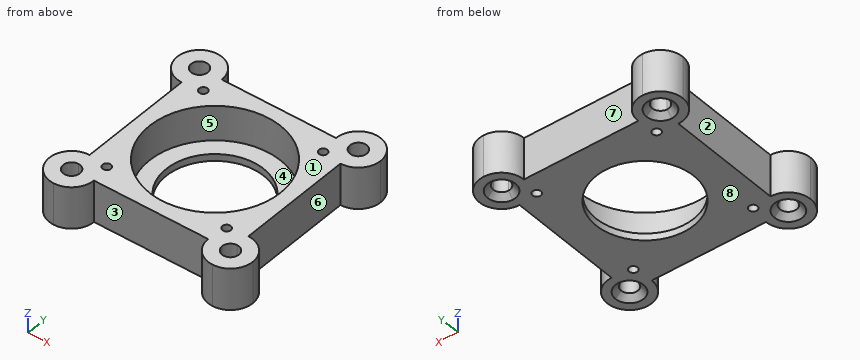
```python
from build123d import *

# Parameters (mm, degrees)
F0_R     = 1.5
F0_R_2   = 23.5
F1_DEPTH = 15
F0_R_3   = 17.5
F2_DEPTH = 2.5
F3_SIZE  = 2


# Not quite as in the source:
# - a feature names something its author has since deleted; it is built from what else it names


with BuildPart() as f1:
    # F0 (on Top) → F1 (new body)
    with BuildSketch(Plane.XY):
        with BuildLine():
            Line((-28.5, 25.5), (-28.5, 20.5))
            ThreePointArc((-28.5, 20.5), (-22.8431457505, 22.8431457505), (-20.5, 28.5))
            Line((-20.5, 28.5), (-25.5, 28.5))
            ThreePointArc((-25.5, 28.5), (-26.3786796564, 26.3786796564), (-28.5, 25.5))
        make_face()
        with BuildLine():
            Line((-20.5, -28.5), (20.5, -28.5))
            ThreePointArc((20.5, -28.5), (22.8431457505, -22.8431457505), (28.5, -20.5))
            Line((28.5, -20.5), (28.5, 20.5))
            ThreePointArc((28.5, 20.5), (22.8431457505, 22.8431457505), (20.5, 28.5))
            Line((20.5, 28.5), (-20.5, 28.5))
            ThreePointArc((-20.5, 28.5), (-22.8431457505, 22.8431457505), (-28.5, 20.5))
            Line((-28.5, 20.5), (-28.5, -20.5))
            ThreePointArc((-28.5, -20.5), (-22.8431457505, -22.8431457505), (-20.5, -28.5))
        make_face()
        with Locations((-21.5, -21.5)):
            Circle(F0_R, mode=Mode.SUBTRACT)
        with Locations((21.5, -21.5)):
            Circle(F0_R, mode=Mode.SUBTRACT)
        with Locations((-21.5, 21.5)):
            Circle(F0_R, mode=Mode.SUBTRACT)
        Circle(F0_R_2, mode=Mode.SUBTRACT)
        with Locations((21.5, 21.5)):
            Circle(F0_R, mode=Mode.SUBTRACT)
        with BuildLine():
            ThreePointArc((20.5, 28.5), (22.8431457505, 22.8431457505), (28.5, 20.5))
            Line((28.5, 20.5), (28.5, 25.5))
            ThreePointArc((28.5, 25.5), (26.3786796564, 26.3786796564), (25.5, 28.5))
            Line((25.5, 28.5), (20.5, 28.5))
        make_face()
        with BuildLine():
            ThreePointArc((28.5, 20.5), (34.1568542495, 22.8431457505), (36.5, 28.5))
            ThreePointArc((36.5, 28.5), (34.1568542495, 34.1568542495), (28.5, 36.5))
            ThreePointArc((28.5, 36.5), (22.8431457505, 34.1568542495), (20.5, 28.5))
            Line((20.5, 28.5), (25.5, 28.5))
            ThreePointArc((25.5, 28.5), (28.5, 31.5), (31.5, 28.5))
            ThreePointArc((31.5, 28.5), (30.6213203436, 26.3786796564), (28.5, 25.5))
            Line((28.5, 25.5), (28.5, 20.5))
        make_face()
        with BuildLine():
            ThreePointArc((20.5, -28.5), (22.8431457505, -34.1568542495), (28.5, -36.5))
            ThreePointArc((28.5, -36.5), (34.1568542495, -34.1568542495), (36.5, -28.5))
            ThreePointArc((36.5, -28.5), (34.1568542495, -22.8431457505), (28.5, -20.5))
            Line((28.5, -20.5), (28.5, -25.5))
            ThreePointArc((28.5, -25.5), (30.6213203436, -26.3786796564), (31.5, -28.5))
            ThreePointArc((31.5, -28.5), (28.5, -31.5), (25.5, -28.5))
            Line((25.5, -28.5), (20.5, -28.5))
        make_face()
        with BuildLine():
            ThreePointArc((28.5, -20.5), (22.8431457505, -22.8431457505), (20.5, -28.5))
            Line((20.5, -28.5), (25.5, -28.5))
            ThreePointArc((25.5, -28.5), (26.3786796564, -26.3786796564), (28.5, -25.5))
            Line((28.5, -25.5), (28.5, -20.5))
        make_face()
        with BuildLine():
            Line((-25.5, -28.5), (-20.5, -28.5))
            ThreePointArc((-20.5, -28.5), (-22.8431457505, -22.8431457505), (-28.5, -20.5))
            Line((-28.5, -20.5), (-28.5, -25.5))
            ThreePointArc((-28.5, -25.5), (-26.3786796564, -26.3786796564), (-25.5, -28.5))
        make_face()
        with BuildLine():
            ThreePointArc((-36.5, -28.5), (-34.1568542495, -34.1568542495), (-28.5, -36.5))
            ThreePointArc((-28.5, -36.5), (-22.8431457505, -34.1568542495), (-20.5, -28.5))
            Line((-20.5, -28.5), (-25.5, -28.5))
            ThreePointArc((-25.5, -28.5), (-30.6213203436, -30.6213203436), (-28.5, -25.5))
            Line((-28.5, -25.5), (-28.5, -20.5))
            ThreePointArc((-28.5, -20.5), (-34.1568542495, -22.8431457505), (-36.5, -28.5))
        make_face()
        with BuildLine():
            ThreePointArc((-28.4999999613, 36.5), (-34.1568542358, 34.1568542632), (-36.5, 28.5))
            ThreePointArc((-36.5, 28.5), (-34.1568542495, 22.8431457505), (-28.5, 20.5))
            Line((-28.5, 20.5), (-28.5, 25.5))
            ThreePointArc((-28.5, 25.5), (-30.6213203436, 30.6213203436), (-25.5, 28.5))
            Line((-25.5, 28.5), (-20.5, 28.5))
            ThreePointArc((-20.5, 28.5), (-22.8431457368, 34.1568542358), (-28.4999999613, 36.5))
        make_face()
    extrude(amount=F1_DEPTH)

    # F0 (on Top) → F2 (join)
    with BuildSketch(Plane.XY):
        Circle(F0_R_2)
        Circle(F0_R_3, mode=Mode.SUBTRACT)
    extrude(amount=F2_DEPTH)

    # F3
    f3_edges = [f1.edges().sort_by_distance(p)[0] for p in [
        (31.5, 28.5, 0),
        (-28.5, 31.5, 0),
        (-31.5, -28.5, 0),
        (28.5, -31.5, 0),
    ]]
    chamfer(f3_edges, length=F3_SIZE)


solid = f1.part
```
Model file for the job. Use its own axes, mm. Face numbers are marked on the shaded views. A direction names the side the tool comes from. Coordinates: 2 decimals unless noted, no trailing zeros. Loops run counter-clockwise (first coordinate to the right, second up) from the corner with the lowest first, then second, coordinate; pieces in that order, holes last. Notation, with made-up numbers: (-6.5, 27) -> (26.5, 27) arc R7 ccw to (26.5, 31) -> close; hole circle Ø3 at (55, 63). An arc over 180 degrees is marked (long way). Answer as a JSON object with one key per item and string values.
Q1. 3-axis set-ups, long thin cutter, end or side, ignore diameter. For the marked faces 5, 6, 7 and 8: which of +Z, -Z, +X, -X, +Y, -Y reach the whole face in a straight line?
Report:
{"face 5": "+Z", "face 6": "+Z, -Z, +X", "face 7": "+Z, -Z, +Y", "face 8": "-Z, +X, -X, +Y, -Y"}
Q2. Cut at A-A (y = 0). List the corners of the cut face in (x, z), and give its area (3 significant figures).
Report:
{"outline": "(-28.5, 0) -> (-17.5, 0) -> (-17.5, 2.5) -> (-23.5, 2.5) -> (-23.5, 15) -> (-28.5, 15) -> close; (17.5, 0) -> (28.5, 0) -> (28.5, 15) -> (23.5, 15) -> (23.5, 2.5) -> (17.5, 2.5) -> close", "area": "180 mm2"}
Q3. Cut at B-B (z = 5.75). State how many separate pieces and enclosed holes the cut face has, and give its area (3 significant figures).
Report:
{"separate pieces": "1", "enclosed holes": "9", "area": "1,980 mm2"}
Q4. Pull direction X, two halves, no side cores. Call the marked faces 1, 2, 3 and 4: released by +X, released by -X, zero draft, split by the parting line, or undercut.
Report:
{"face 1": "zero draft", "face 2": "released by -X", "face 3": "undercut", "face 4": "undercut"}
Q5. Probe probe 1 along Y at (x, z) = (21.5, 3.25); probe 2 along X at (y, z) = (-28, 2.25); probe 3 along X at (y, z) = (29.5, 8.25). List the from-to ranges inside material, lowest first.
Report:
{"probe 1": "y = -32.37 to -23, -20 to -9.49, 9.49 to 20, 23 to 32.37", "probe 2": "x = -36.48 to -31.46, -25.54 to 25.54, 31.46 to 36.48", "probe 3": "x = -36.44 to -31.33, -25.67 to -20.56, 20.56 to 25.67, 31.33 to 36.44"}
Q6. Flat gauge pins, fed straight in: P1, Ø10, axis at x = 3.5, y = -9, coming from the -Z side; P2, Ø2, axis at y = -16, z = 10, coming from the -X side; P3, Ø8, axis at x = -28.5, y = 28.5, coming from the -Z side; P4, Ø7.5, axis at x = 1.5, z = 6, coming from the -Y side. Where does each tip first touch, or does it go through?
Report:
{"P1": "passes through", "P2": "stops at x = -28.5", "P3": "stops at z = 1", "P4": "stops at y = -28.5"}
Q7. Cut at D-D (x = 19). List the corners of the cut face in (y, z).
Report:
{"outline": "(-28.5, 0) -> (28.5, 0) -> (28.5, 15) -> (13.83, 15) -> (13.83, 2.5) -> (-13.83, 2.5) -> (-13.83, 15) -> (-28.5, 15) -> close"}
